Autodesk Inventor part; units mm, degrees
ref_plane "YZ Plane" through (0, 0, 0) normal (1, 0, 0) x (0, 1, 0)
ref_plane "XZ Plane" through (0, 0, 0) normal (0, 1, 0) x (-1, 0, 0)
ref_plane "XY Plane" through (0, 0, 0) normal (0, 0, 1) x (1, 0, 0)
sketch "Sketch1" plane through (0, 0, 0) normal (0, 1, 0) x (-1, 0, 0)
  circle A0 centre (0, 0) radius 7.925
  dimension "d5" = 15.85
extrude "Extrusion1" add sketch "Sketch1" along normal blind 16
sketch "Sketch2" plane through (0, 0, 0) normal (1, 0, 0) x (0, 1, 0)
  line L0 (16, -7.925) -> (16, 7.925)
  line L1 (0, 7.925) -> (0, -7.925)
  line L2 (0, 7.925) -> (0, -7.925)
  line L3 (0, 7.925) -> (-21.5, 0)
  line L4 (-21.5, 0) -> (0, 0)
  line L5 (0, 7.925) -> (0, 0)
  dimension "d2" = 21.5
revolve "Revolution1" add sketch "Sketch2" angle 360 about axis through (0, -21.5, 0) along (0, 1, 0)
shell "Shell1" thickness 1 removed faces 1 at (2.2031, 16, 0.1081)
properties part number "FalconTube15mL"
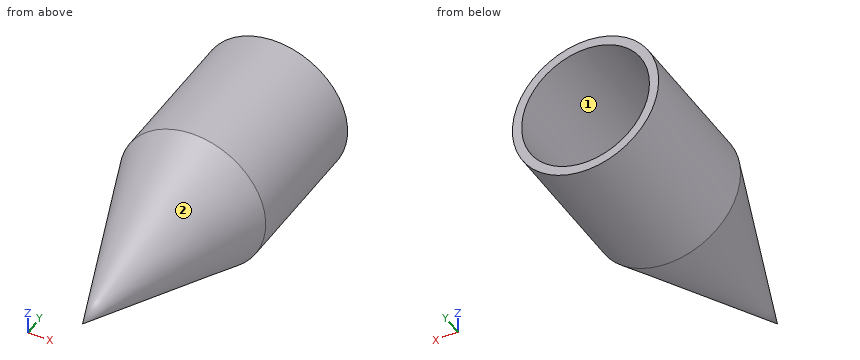
Can you work these out from the model? Positions are in its coordinate system, mm. Face numbers are marked on the shaded views. Coordinates: 2 decimals unless noted, no trailing zeros. Loops run counter-clockwise (first coordinate to the right, second up) from the corner with the lowest first, then second, coordinate; pieces in that order, holes last. Notation, with made-up numbers: M 59.5,28.25 L 76.5,28.25 A18 ccw 76.5,32.25 Z; hole C -33,46 d4. An arc over 180 degrees is marked long. Answer as CSV lines item,"result". Start each with the question number.
1. If I drill on probe 1 along X at (y, z) = (12, 0) (3 decimals); probe 2 along X at (y, z) = (4, -4.25), over which ranges is the centre line in solid material (lowest first)? Write a range as [from, to].
2. Suppose I cut it at B-B, the plane y = -13. List the corners of the cut face in (x, z) for me, plus the area to 3 significant figures.
3. For pin 1 Ø6 at (y, z) = (-13, -5.5) entering from +X; pin 2 Ø2 at (x, y) = (1, -10) entering from +Z; pin 3 Ø1.5 at (y, z) = (-5.5, -4.5) entering from -X, each with a flat end and sliding along its axis, tell me the tip position at first contact or that it passes through.
4. Suppose I cut it at A-A, the plane y = -3. List the corners of the cut face in (x, z) for me.
5. Thinking about a two-plate mould opening in Z: for the marked faces 1 and 2, which applies, +Z half, -Z half, draft (parallel to the pull), parting line (faces both ways), or undercut?
Output:
1,probe 1,"x = [-7.925, -6.925], [6.925, 7.925]"
1,probe 2,"x = [-6.69, -5.47], [5.47, 6.69]"
2,outline,"C 0,0 d6.27; hole C 0,0 d4.13"
2,area,"17.4 mm^2"
3,pin 1,"stops at x = 2.29"
3,pin 2,"stops at z = 4.54"
3,pin 3,"stops at x = -4.65"
4,outline,"C 0,0 d13.64; hole C 0,0 d11.51"
5,face 1,"undercut"
5,face 2,"parting line"
